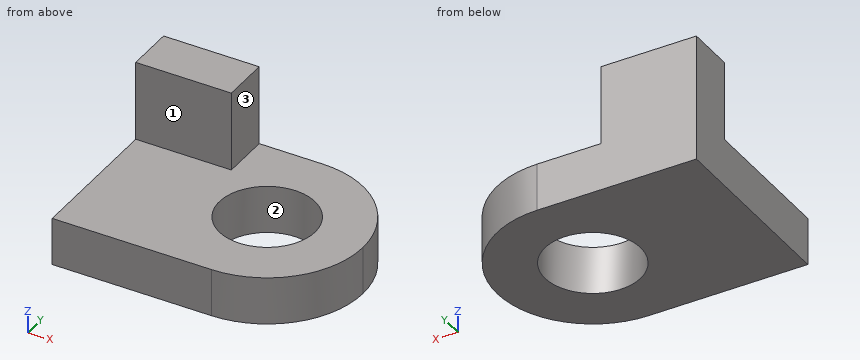
from build123d import *

# Parameters (mm, degrees)
F0_R     = 21
F1_DEPTH = 21
F2_W     = 42
F2_H     = 21
F3_DEPTH = 35


with BuildPart() as f1:
    # F0 (on Top) → F1 (new body)
    with BuildSketch(Plane.XY):
        with BuildLine():
            Line((14, 42), (-56, 42))
            Line((-56, 42), (-56, -42))
            Line((-56, -42), (14, -42))
            ThreePointArc((14, -42), (43.698485, -29.698485), (56, 0))
            ThreePointArc((56, 0), (43.698485, 29.698485), (14, 42))
        make_face()
        with Locations((14, 0)):
            Circle(F0_R, mode=Mode.SUBTRACT)
    extrude(amount=F1_DEPTH)

    # F2 (on face) → F3 (join)
    with BuildSketch(Plane.XY.offset(21)):
        with Locations((-35, 31.5)):
            Rectangle(F2_W, F2_H)
    extrude(amount=F3_DEPTH)


solid = f1.part
Check sheet for the modelled part. Datum: model origin and axes. Units: mm. Face numbers are marked on the shaded views. Round coordinates to 2 decimals unless told otherwise and drop trailing zeros. Order: outer loops, then holes, each group sorted by start corner. A loop starts at its lowest first (then second) coordinate and runs counter-clockwise, first axis right, second up. Notation, with made-up numbers: M -15,-36.75 L 33,-36.75 A35 cw 33,-4.75 Z; hole C -35,-11.75 d5. An arc over 180 degrees is marked long. One line per item, written item: value. Start each with the question number.
1. Section check D-D on x = -49. Enter the section's corners in (y, z).
2. Release check for a two-part mould opening along Y. For the marked faces 1, 2 and 3 record: released by +Y, released by -Y, zero draft, split by the parting line, or undercut.
3. Gauge pin test, flat ends, axial feed: P1, Ø6.5, axis at y = 28, z = 41.5, coming from the +X side; P2, Ø25, axis at x = -21, y = 3.5, coming from the +Z side. Record the tip position at first contact, or that the pin passes through.
4. Scan lines: line 1 along Z through (x, y) = (5, 31.5); line 2 along Y through (x, z) = (15.5, 4); line 3 along X through (y, z) = (32, 51.5). Record each from-to range of solid material in increasing order.
5. Section check C-C on x = -5. Enter the section's corners in (y, z), and give its area (3 significant figures).
6. Section check A-A on y = -1.5. Enter the section's corners in (x, z), and give its area (3 significant figures).
7. Section check B-B on z = 13.5. Enter the section's corners in (x, y), and give its area (3 significant figures).
Results found:
1. outline: M -42,0 L 42,0 L 42,56 L 21,56 L 21,21 L -42,21 Z
2. face 1: released by -Y
2. face 2: undercut
2. face 3: zero draft
3. P1: x = -14
3. P2: z = 21
4. line 1: 0 to 21
4. line 2: -41.97 to -20.95, 20.95 to 41.97
4. line 3: -56 to -14
5. outline: M -42,0 L -8.94,0 L -8.94,21 L -42,21 Z; M 8.94,0 L 42,0 L 42,21 L 8.94,21 Z
5. area: 1,390 mm^2
6. outline: M -56,0 L -6.95,0 L -6.95,21 L -56,21 Z; M 34.95,0 L 55.97,0 L 55.97,21 L 34.95,21 Z
6. area: 1,470 mm^2
7. outline: M -56,-42 L 14,-42 A42 ccw 56,0 A42 ccw 14,42 L -56,42 Z; hole C 14,0 d42
7. area: 7,270 mm^2
